For this review, take the finished solid that the model builds, in its own axes (mm). Give positions to 0.01 mm unless a question says otherwise; leave off trailing zeros. Loops run counter-clockwise (first coordinate to the right, second up) from the corner with the lowest first, then second, coordinate; pieces in that order, holes last. Notation, with made-up numbers: (86, 52.5) -> (132, 52.5) arc R16 cw to (132, 66.5) -> close; hole circle Ø4 at (10.5, 45.5). An arc over 180 degrees is marked (long way). Answer as CSV lines item,"result". Start each with the question number.
Item 1: Add section C-C on y = 0.7. State the section outline as (x, z) points, plus the area to 3 significant figures.
Item 2: For L1, parallel to Z at x = 0, y = 0.35; L2, parallel to X at y = 0.35, z = 0; L3, parallel to X at y = 0.1, z = 10.75, list the stretches that pass through material, from the lowest coordinate up. Write a range as from..to.
Item 3: Add section A-A on x = -8. State the section outline as (y, z) points.
Item 4: Add section B-B on z = 6.5. State the section outline as (x, y) points, plus the area to 3 significant figures.
```python
from build123d import *

# Parameters (mm, degrees)
SKETCH1_R               = 12.7
SKETCH1_R_2             = 11.8745
BOSS_EXTRUDE1_DEPTH     = 1.016
CUT_EXTRUDE1_REACH      = 19.989
CUT_EXTRUDE1_END_RADIUS = 12.7


with BuildPart() as part:
    # Sketch1 → Boss-Extrude1 (new body)
    with BuildSketch(Plane(origin=(0, 0, 0), x_dir=(1, 0, 0), z_dir=(0, 1, 0))):
        with Locations(Location((0, 0, 0), (0, 0, 270))):
            Circle(SKETCH1_R)
        with Locations(Location((0, 0, 0), (0, 0, 270))):
            Circle(SKETCH1_R_2, mode=Mode.SUBTRACT)
    extrude(amount=BOSS_EXTRUDE1_DEPTH)

    # Cut-Extrude1: up to this cylinder (the profile starts inside it)
    cut_extrude1_end = Plane(origin=(0, 0.508, 0), z_dir=(0, -1, 0)) * Cylinder(CUT_EXTRUDE1_END_RADIUS, 66.378, mode=Mode.PRIVATE)
    # Sketch2 → Cut-Extrude1 (cut, up to the surface)
    with BuildSketch(Plane(origin=(0, 0, 0), x_dir=(0, 0, -1), z_dir=(1, 0, 0)), mode=Mode.PRIVATE) as cut_extrude1_sk1:
        Polygon((0, 0), (1.016, 1.016), (-0.420840979, 1.016), (-1.436840979, 0), align=None)
    cut_extrude1_tool1 = extrude(cut_extrude1_sk1.sketch, amount=-CUT_EXTRUDE1_REACH, mode=Mode.PRIVATE) & cut_extrude1_end
    add(cut_extrude1_tool1.solids().sort_by_distance((0, 0.508, 0.21042))[0], mode=Mode.SUBTRACT)


solid = part.part
```
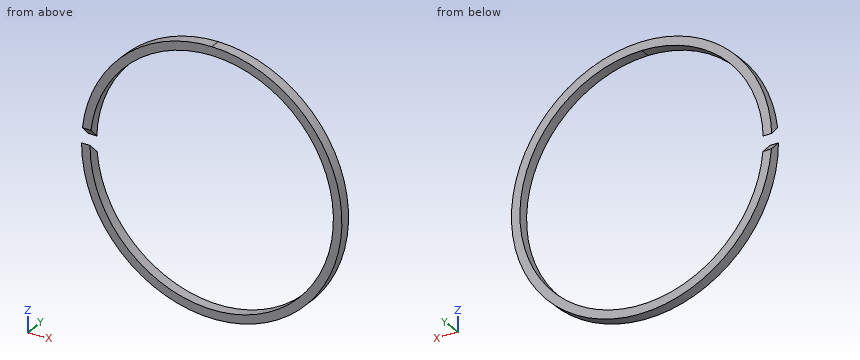
Computed values:
1,outline,"(-12.68, -0.7) arc R12.7 ccw (long way) to (-12.68, 0.74) -> (-11.85, 0.74) arc R11.87 cw (long way) to (-11.85, -0.7) -> close"
1,area,"62.5 mm²"
2,L1,"-12.7..-11.87, 11.87..12.7"
2,L2,"11.87..12.7"
2,L3,"-6.76..-5.04, 5.04..6.76"
3,outline,"(0, -9.86) -> (1.02, -9.86) -> (1.02, -8.78) -> (0, -8.78) -> close; (0, 8.78) -> (1.02, 8.78) -> (1.02, 9.86) -> (0, 9.86) -> close"
4,outline,"(-10.91, 0) -> (-9.94, 0) -> (-9.94, 1.02) -> (-10.91, 1.02) -> close; (9.94, 0) -> (10.91, 0) -> (10.91, 1.02) -> (9.94, 1.02) -> close"
4,area,"1.98 mm²"
